Input: part model. Units: mm. Frame: model coordinates. Face numbers are marked on the shaded views. A direction names the side the tool comes from. Coordinates: 2 decimals unless noted, no trailing zeros. Order: outer loops, then holes, each group sorted by start corner. A loop starts at its lowest first (then second) coordinate and runs counter-clockwise, first axis right, second up. Notation, with made-up numbers: (46.25, 39) -> (55.25, 39) arc R36 ccw to (55.25, 73) -> close; hole circle Ø9 at (-5, 85.5). An arc over 180 degrees is marked (long way). Answer as CSV lines item,"result".
from build123d import *

# Parameters (mm, degrees)
F2_R     = 8
F3_DEPTH = 2


with BuildPart() as f1:
    # F0 (on Right) → F1 (revolve)
    with BuildSketch(Plane.YZ):
        Polygon((-23.5, 0), (0, 0), (0, 3), (-5, 3), (-5, 3.5), (-6.5, 3.5), (-8, 7), (-8, 8.8), (-16.5, 8.8), (-19, 5), (-19, 2.5), (-19.5, 2.5), (-19.5, 1), (-23.5, 1), align=None)
    revolve(axis=Axis((0, -11.75, 0), (0, 1, 0)))

    # F2 (on face) → F3 (cut)
    with BuildSketch(Plane.XZ.offset(19)):
        with Locations((0, 11)):
            Circle(F2_R)
        with Locations((-9.526279, -5.5)):
            Circle(F2_R)
        with Locations((9.526279, -5.5)):
            Circle(F2_R)
    extrude(amount=-F3_DEPTH, mode=Mode.SUBTRACT)


solid = f1.part
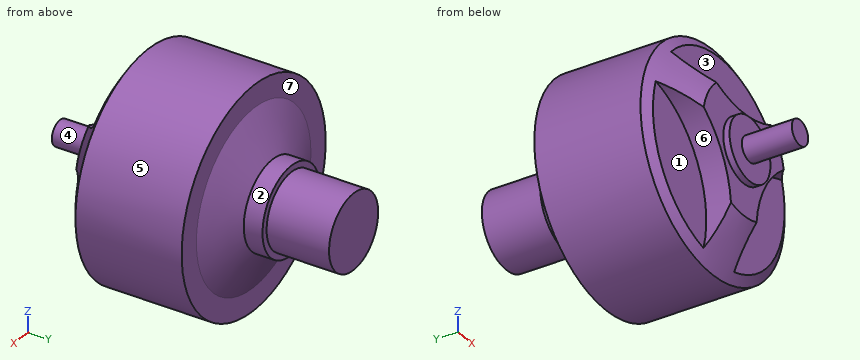
1. Cut plane D-D (y = -2.75). Return the cut outline in (x, z).
Findings:
outline,"circle Ø6 at (0, 0)"
2. Cut plane A-A (x = 0). Return the cut outline in (y, z).
Findings:
outline,"(-23.5, -1) -> (-19.5, -1) -> (-19.5, -2.5) -> (-19, -2.5) -> (-19, -5) -> (-16.5, -8.8) -> (-8, -8.8) -> (-8, -7) -> (-6.5, -3.5) -> (-5, -3.5) -> (-5, -3) -> (0, -3) -> (0, 3) -> (-5, 3) -> (-5, 3.5) -> (-6.5, 3.5) -> (-8, 7) -> (-8, 8.8) -> (-16.5, 8.8) -> (-17, 8.04) -> (-17, 3) -> (-19, 3) -> (-19, 2.5) -> (-19.5, 2.5) -> (-19.5, 1) -> (-23.5, 1) -> close"
3. Reachability of the marked faces 4, 5, 6 and 7 from +Z, -Z, +X, -X, +Y, -Y: full face, straight path, thin tool, end or side. Return the list, or none.
Findings:
face 4,"-Y"
face 5,"+Y, -Y"
face 6,"-X, -Y"
face 7,"+Y"
4. Contact query for flat-ended pins moving along their axis: pin 1 (1.5 mm diameter, centred on x = -3, z = 6.5, fed in from -Y); pin 2 (5 mm diameter, centred on x = -4.5, z = -1, fed in from -Y); pin 3 (4 mm diameter, centred on x = 2.5, y = -17, fed in from -Z); pin 4 (4 mm diameter, centred on x = -7, y = -20.5, fed in from +Z). Output: stop coordinate, or through.
Findings:
pin 1,"stops at y = -17"
pin 2,"stops at y = -19.5"
pin 3,"stops at z = -8.78"
pin 4,"passes through"
5. Cut plane B-B (z = 0). Return the cut outline in (x, y).
Findings:
outline,"(-8.8, -16.5) -> (-8.04, -17) -> (-3.72, -17) -> (-3.72, -19) -> (-2.5, -19) -> (-2.5, -19.5) -> (-1, -19.5) -> (-1, -23.5) -> (1, -23.5) -> (1, -19.5) -> (2.5, -19.5) -> (2.5, -19) -> (3.72, -19) -> (3.72, -17) -> (8.04, -17) -> (8.8, -16.5) -> (8.8, -8) -> (7, -8) -> (3.5, -6.5) -> (3.5, -5) -> (3, -5) -> (3, 0) -> (-3, 0) -> (-3, -5) -> (-3.5, -5) -> (-3.5, -6.5) -> (-7, -8) -> (-8.8, -8) -> close"
6. Ray query, line 1 along Y through (x, z) = (-1.25, -2); line 2 along X through (y, z) = (-1, 0); line 3 along Y through (x, z) = (-2.75, -0.5). Return the intervals inside material, ascending.
Findings:
line 1,"y = -19.5 to 0"
line 2,"x = -3 to 3"
line 3,"y = -19 to 0"
7. Mould query, pull axis X, two halves, no side actions, for the marked faces 1, 2 and 3. Classes: released by +X, released by -X, zero draft, split by the parting line, or undercut.
Findings:
face 1,"zero draft"
face 2,"split by the parting line"
face 3,"undercut"
8. Cut plane C-C (y = -11.75). Return the cut outline in (x, z), plus the area to 3 significant figures.
Findings:
outline,"circle Ø17.6 at (0, 0)"
area,"243 mm2"
